from build123d import *

# Parameters (mm, degrees)
LONG_LEG_W             = 30
LONG_LEG_H             = 150
LONG_LEG_EXTRUDE_DEPTH = 10
SKETCH2_W              = 30
SKETCH2_H              = 30
BOSS_EXTRUDE2_DEPTH    = 10
SKETCH6_W              = 15
SKETCH6_H              = 10
LONG_LEG_DOWN_DEPTH    = 20
SKETCH12_W             = 20
SKETCH12_H             = 30
BOSS_EXTRUDE8_DEPTH    = 10
SKETCH13_W             = 6
SKETCH13_H             = 5
CUT_EXTRUDE2_DEPTH     = 10
FILLET1_R              = 2
FILLET2_R              = 2
FILLET3_R              = 2
FILLET4_R              = 2


with BuildPart() as part:
    # long-leg → long_leg_extrude (new body)
    with BuildSketch(Plane(origin=(0, 0, 0), x_dir=(0, 1, 0), z_dir=(0, 0, 1))):
        with Locations((-2.514124294, -68.610169492)):
            Rectangle(LONG_LEG_W, LONG_LEG_H)
    extrude(amount=LONG_LEG_EXTRUDE_DEPTH)

    # Sketch2 → Boss-Extrude2 (add)
    with BuildSketch(Plane(origin=(-6.389830508, 0, 0), x_dir=(0, -1, 0), z_dir=(-1, 0, 0))):
        with Locations((2.514124294, -5)):
            Rectangle(SKETCH2_W, SKETCH2_H)
    extrude(amount=BOSS_EXTRUDE2_DEPTH)

    # Sketch6 → long leg down (add)
    with BuildSketch(Plane.XZ.offset(17.514124294)):
        Polygon((-6.389830508, 0), (-6.389830508, 10), (-16.389830508, 10), (-16.389830508, -20), (-6.389830508, -20), align=None)
        Polygon((8.610169492, 0), (-6.389830508, 0), (-6.389830508, -20), (-6.389830508, -190), (8.610169492, -190), align=None)
        with Locations((1.110169492, 5)):
            Rectangle(SKETCH6_W, SKETCH6_H)
    extrude(amount=LONG_LEG_DOWN_DEPTH)

    # Sketch12 → Boss-Extrude8 (add)
    with BuildSketch(Plane(origin=(0, 12.485875706, 0), x_dir=(-1, 0, 0), z_dir=(0, 1, 0))):
        with Locations((-133.610169492, -5)):
            Rectangle(SKETCH12_W, SKETCH12_H)
    extrude(amount=BOSS_EXTRUDE8_DEPTH)

    # Sketch13 → Cut-Extrude2 (cut)
    with BuildSketch(Plane(origin=(-6.389830508, 0, 0), x_dir=(0, -1, 0), z_dir=(-1, 0, 0))):
        Polygon((24.559120017, -185), (30.559120017, -185), (33.559120017, -185), (33.559120017, -180), (21.559120017, -180), (21.559120017, -185), align=None)
        with Locations((27.559120017, -187.5)):
            Rectangle(SKETCH13_W, SKETCH13_H)
    extrude(amount=-CUT_EXTRUDE2_DEPTH, mode=Mode.SUBTRACT)

    # Fillet1
    fillet1_edges = [part.edges().sort_by_distance(p)[0] for p in [
        (133.610169492, 12.485875706, -20),
        (133.610169492, 22.485875706, -20),
        (133.610169492, 22.485875706, 10),
        (143.610169492, 2.485875706, 10),
        (-16.389830508, -12.514124294, 10),
        (-16.389830508, -12.514124294, -20),
    ]]
    fillet(fillet1_edges, radius=FILLET1_R)

    # Fillet2
    fillet2_edges = [part.edges().sort_by_distance(p)[0] for p in [
        (143.610169492, -17.514124294, 4),
        (143.024383054, -17.514124294, 9.414213562),
        (75.110169492, -17.514124294, 10),
        (8.610169492, -37.514124294, -90),
        (8.610169492, -27.514124294, 10),
        (-6.389830508, -37.514124294, -105),
        (143.610169492, -2.514124294, 0),
    ]]
    fillet(fillet2_edges, radius=FILLET2_R)

    # Fillet3
    fillet3_edges = [part.edges().sort_by_distance(p)[0] for p in [
        (8.610169492, -17.514124294, -95),
    ]]
    fillet(fillet3_edges, radius=FILLET3_R)

    # Fillet4
    fillet4_edges = [part.edges().sort_by_distance(p)[0] for p in [
        (-16.389830508, 12.485875706, -5),
        (-10.389830508, 12.485875706, -20),
        (-15.804044071, 12.485875706, -19.414213562),
        (-15.804044071, 12.485875706, 9.414213562),
        (54.610169492, 12.485875706, 10),
    ]]
    fillet(fillet4_edges, radius=FILLET4_R)


solid = part.part
Could you check a few things on this model? Use its own coordinates, in mm. A direction names the side the tool comes from. Round coordinates to 2 decimals unless told otherwise and drop trailing zeros. Write each loop counter-clockwise with the first axis right and the second up, starting at its lowest first coordinate (ties: lowest second). Pieces come first, ordered by that corner, then holes. Notation, with made-up numbers: (86, 10) - (120, 10) arc R12 ccw to (120, 29) - close; hole circle Ø11 at (78.25, 72). An arc over 180 degrees is marked (long way). Put each result on its own line as item: value. Start each with the question number.
(1) I want a section at D-D, the plane z = -36. Please give me the cut outline in (x, y).
(2) I need wall thicknesses on probe 1 along Z at (x, y) = (21, -5); probe 2 along X at (y, z) = (-28, -61); probe 3 along Y at (x, z) = (0, -171.5). Which ranges of each line are inside material? Lowest first, please.
(3) Thinking about a two-plate mould opening in Y: for faces 6 (the flat face through (123.61, 18, -5)), 7 (the flat face through (0, -37.514, -89)), 8 (the flat face through (3.61, -27, -184)), which applies, released by +Y, released by -Y, zero draft, split by the parting line, or undercut?
(4) Will these pins go through, and if not, where does the flat tip stop? pin 1 (22 mm diameter, centred on x = 134.5, z = -11.5, fed in from -Y); pin 2 (21 mm diameter, centred on x = 52, z = -7.5, fed in from +Y); pin 3 (5 mm diameter, centred on y = -28.5, z = -114, fed in from -X); pin 4 (8 mm diameter, centred on x = -3, y = -25, fed in from -Z).
(5) I want a section at A-A, the plane z = -15. Please give me the cut outline in (x, y), plus the area to 3 significant figures.
(6) I want a section at B-B, the plane y = -3. Please give me the cut outline in (x, z).
(7) I want a section at C-C, the plane x = 0. Please give me the cut outline in (y, z), plus the area to 3 significant figures.
(8) For faces 1 (the flat face through (-6.39, -26, -104)), 2 (the flat face through (-1, -33.559, -183)), 3 (the flat face through (45, 12.486, 2)), 4 (the flat face through (-6.39, -2, -10)), 5 (the flat face through (-1, -30.559, -188)), which set-ups out of +Z, -Z, +X, -X, +Y, -Y let a thin tool reach every point of the face, with its end or its side?
Here are the results:
1. outline: (-6.39, -35.51) arc R2 ccw to (-4.39, -37.51) - (6.61, -37.51) arc R2 ccw to (8.61, -35.51) - (8.61, -19.51) arc R2 ccw to (6.61, -17.51) - (-6.39, -17.51) - close
2. probe 1: z = 0 to 10
2. probe 2: x = -6.39 to 8.61
2. probe 3: y = -37.51 to -17.51
3. face 6: zero draft
3. face 7: released by -Y
3. face 8: undercut
4. pin 1: stops at y = 12.49
4. pin 2: stops at y = 12.49
4. pin 3: stops at x = -6.39
4. pin 4: stops at z = -190
5. outline: (-16.39, -37.51) - (6.61, -37.51) arc R2 ccw to (8.61, -35.51) - (8.61, -19.51) arc R2 ccw to (6.61, -17.51) - (-6.39, -17.51) - (-6.39, 12.49) - (-14.39, 12.49) arc R2 ccw to (-16.39, 10.49) - close; (123.61, 12.49) - (143.61, 12.49) - (143.61, 22.49) - (123.61, 22.49) - close
5. area: 997 mm^2
6. outline: (-16.39, -18) arc R2 ccw to (-14.39, -20) - (-6.39, -20) - (-6.39, 0) - (141.61, 0) arc R2 ccw to (143.61, 2) - (143.61, 8) arc R2 ccw to (141.61, 10) - (-14.39, 10) arc R2 ccw to (-16.39, 8) - close
7. outline: (-37.51, -190) - (-30.56, -190) - (-30.56, -185) - (-33.56, -185) - (-33.56, -180) - (-21.56, -180) - (-21.56, -185) - (-24.56, -185) - (-24.56, -190) - (-17.51, -190) - (-17.51, 0) - (12.49, 0) - (12.49, 8) arc R2 ccw to (10.49, 10) - (-37.51, 10) - close
7. area: 4,210 mm^2
8. face 1: -Z, -X, +Y, -Y
8. face 2: -X
8. face 3: +Z, -Z, -X, +Y
8. face 4: -Z, +X, +Y
8. face 5: -Z, -X
